Can you work these out from the model? Positions are in its coordinate system, mm. Coordinates: 2 decimals unless noted, no trailing zeros. Write each loop counter-clockwise with the first axis right and the second up, starting at its lowest first coordinate (ties: lowest second). Pieces come first, ordered by that corner, then holes. Notation, with made-up numbers: M 86,-35.5 L 104,-35.5 A23 ccw 104,-27.5 Z; hole C -35.75,25.25 d8. An arc over 180 degrees is marked long. Answer as a JSON object with one key per item and string values. Group by question number.
from build123d import *

# Parameters (mm, degrees)
F0_R     = 6
F1_DEPTH = 750
F3_DEPTH = 600


with BuildPart() as f1:
    # F0 (on Front) → F1 (new body, symmetric)
    with BuildSketch(Plane.XZ):
        Circle(F0_R)
    extrude(amount=F1_DEPTH, both=True)

    # F2 (on Front) → F3 (join, symmetric)
    with BuildSketch(Plane.XZ):
        with BuildLine():
            Line((-55, 26.90525), (-58.4375, 23.274328))
            ThreePointArc((-58.4375, 23.274328), (0, 0), (58.4375, 23.274328))
            Line((58.4375, 23.274328), (55, 26.90525))
            ThreePointArc((55, 26.90525), (0, 5), (-55, 26.90525))
        make_face()
    extrude(amount=F3_DEPTH, both=True)


solid = f1.part
Q1. If we section it at A-A on y = 166: List the corners of the cut face in (x, z) for me, and give its area (3 significant figures).
Q2. Will these pins go through, and if not, where does the flat tip stop? pin 1 (12 mm diameter, centred on x = -23.5, y = -56, fed in from -Z); pin 2 (13.5 mm diameter, centred on x = -22.5, z = 17.5, fed in from +Y); pin 3 (1 mm diameter, centred on x = -30, y = 587, fed in from +Z); pin 4 (8 mm diameter, centred on x = 18.5, z = 9, fed in from +Y).
Q3. We'd pull the mould along X, two halves only. Please class faces 1 (the cylindrical face through (-34.592, -8.4, 7.357)), 2 (the cylindrical face through (-30.719, -8.4, 11.133)), 3 (the flat face through (31, -600, 11)), 4 (the cylindrical face through (33.844, -8.4, 7.028)): pulls with the +X half, pulls with the -X half, needs draft (parallel to the pull), parting line crosses it, or undercut.
Q4. If we section it at B-B on z = 12.5: List the corners of the cut face in (x, y) for me.
Q5. If we section it at C-C on x = -38: List the corners of the cut face in (y, z) for me, and give its area (3 significant figures).
Q6. If we section it at D-D on x = 19: List the corners of the cut face in (y, z) for me, and give its area (3 significant figures).
Q7. Please list where these lines run through material, in increasing order: L1, parallel to Y at x = -12, z = 4; L2, parallel to X at y = 254.5, z = 12; L3, parallel to Z at x = 14.5, y = 466.
Reply:
{
 "1": {"outline": "M -58.44,23.27 A85 ccw -6,0.21 A6 ccw long 6,0.21 A85 ccw 58.44,23.27 L 55,26.91 A80 cw 3.22,5.06 A6 ccw -3.22,5.06 A80 cw -55,26.91 Z", "area": "687 mm^2"},
 "2": {"pin 1": "z = 1.82", "pin 2": "through", "pin 3": "z = 11.04", "pin 4": "y = 600"},
 "3": {"face 1": "pulls with the -X half", "face 2": "undercut", "face 3": "needs draft", "face 4": "pulls with the +X half"},
 "4": {"outline": "M -44.37,-600 L -33.82,-600 L -33.82,600 L -44.37,600 Z; M 33.82,-600 L 44.37,-600 L 44.37,600 L 33.82,600 Z"},
 "5": {"outline": "M -600,8.97 L 600,8.97 L 600,14.6 L -600,14.6 Z", "area": "6,760 mm^2"},
 "6": {"outline": "M -600,2.15 L 600,2.15 L 600,7.29 L -600,7.29 Z", "area": "6,170 mm^2"},
 "7": {"L1": "-600 to 600", "L2": "-43.54 to -32.73, 32.73 to 43.54", "L3": "1.25 to 6.33"}
}
